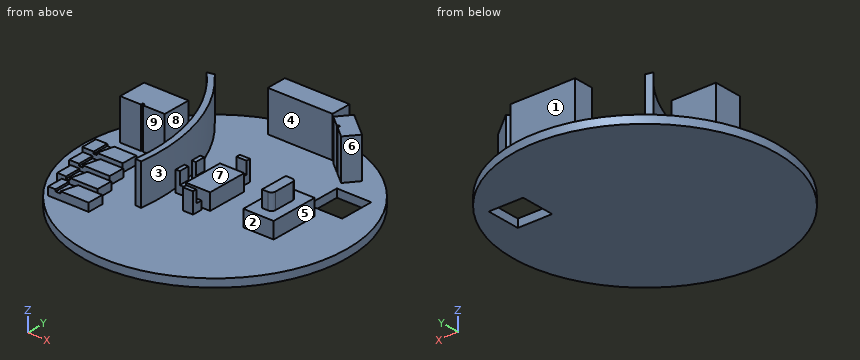
```python
from build123d import *

# Parameters (mm, degrees)
F0_R      = 32.5
F1_DEPTH  = 2
F2_W      = 16
F2_H      = 5
F3_DEPTH  = 10
F4_W      = 6
F4_H      = 10
F4_W_2    = 7.5
F4_H_2    = 12
F5_DEPTH  = 4
F6_W      = 2.5
F6_H      = 7
F7_DEPTH  = 4
F8_R      = 1
F9_W      = 2.5
F9_H      = 2.5
F10_DEPTH = 2
F11_W     = 2.5
F11_H     = 1
F11_W_2   = 1
F11_H_2   = 2.5
F12_DEPTH = 3
F13_W     = 8.5
F13_H     = 8.5
F14_DEPTH = 25
F15_W     = 10
F15_H     = 4
F16_DEPTH = 1.5
F17_W     = 2.795801
F17_H     = 4
F17_W_2   = 2.404703
F17_W_3   = 2.193978
F17_W_4   = 1.803281
F18_DEPTH = 0.5


with BuildPart() as f1:
    # F0 (on Top) → F1 (new body)
    with BuildSketch(Plane.XY):
        Circle(F0_R)
    extrude(amount=F1_DEPTH)

    # F2 (on face) → F3 (join)
    with BuildSketch(Plane.XY.offset(2)):
        with Locations((-0.270834, 27.762719)):
            Rectangle(F2_W, F2_H)
        Polygon((17.300418, 22.562942), (11.08706, 27.602206), (8.567428, 24.495527), (11.384874, 22.210474), (11.699828, 22.598809), (12.088162, 22.283855), (11.773208, 21.89552), (14.780786, 19.456263), align=None)
        Polygon((-16.460359, 11.750014), (-27.460359, 11.750014), (-27.460359, 4.750014), (-22.328375, 4.750014), (-22.328375, 5.250014), (-21.828375, 5.250014), (-21.828375, 4.750014), (-16.460359, 4.750014), align=None)
        with BuildLine():
            Line((-9.214541, -12.358905), (-7.719307, -12.482575))
            ThreePointArc((-7.719307, -12.482575), (-9.766223, 6.462552), (-19.395168, 22.906126))
            Line((-19.395168, 22.906126), (-21.053303, 22.485526))
            ThreePointArc((-21.053303, 22.485526), (-11.314103, 6.361134), (-9.214541, -12.358905))
        make_face()
    extrude(amount=F3_DEPTH)

    # F4 (on face) → F5 (join)
    with BuildSketch(Plane.XY.offset(2)):
        Rectangle(F4_W, F4_H)
        with Locations((15.75, 0.081453)):
            Rectangle(F4_W_2, F4_H_2)
    extrude(amount=F5_DEPTH)

    # F6 (on face) → F7 (join)
    with BuildSketch(Plane.XY.offset(6)):
        with Locations((15.75, 0.081453)):
            Rectangle(F6_W, F6_H)
    extrude(amount=F7_DEPTH)

    # F8
    f8_edges = [f1.edges().sort_by_distance(p)[0] for p in [
        (17, -3.418547, 8),
        (17, 3.581453, 8),
    ]]
    fillet(f8_edges, radius=F8_R)

    # F9 (on face) → F10 (join)
    with BuildSketch(Plane.XY.offset(2)):
        with Locations((-5.362472, -2.423183)):
            Rectangle(F9_W, F9_H)
        with Locations((-5.374835, 2.296795)):
            Rectangle(F9_W, F9_H)
        with Locations((0.118701, 7.372063)):
            Rectangle(F9_W, F9_H)
        with Locations((0.21179, -6.925349)):
            Rectangle(F9_W, F9_H)
    extrude(amount=F10_DEPTH)

    # F11 (on face) → F12 (join)
    with BuildSketch(Plane.XY.offset(4)):
        with Locations((0.21179, -7.675349)):
            Rectangle(F11_W, F11_H)
        with Locations((-6.124835, 2.296795)):
            Rectangle(F11_W_2, F11_H_2)
        with Locations((-6.112472, -2.423183)):
            Rectangle(F11_W_2, F11_H_2)
        with Locations((0.118701, 8.122063)):
            Rectangle(F11_W, F11_H)
    extrude(amount=F12_DEPTH)

    # F13 (on face) → F14 (cut)
    with BuildSketch(Plane.XY.offset(2)):
        with Locations((19.782292, 13.050183)):
            Rectangle(F13_W, F13_H)
    extrude(amount=-F14_DEPTH, mode=Mode.SUBTRACT)

    # F15 (on face) → F16 (join)
    with BuildSketch(Plane.XY.offset(2)):
        with Locations((-24.43407, -2)):
            Rectangle(F15_W, F15_H)
        with Locations((-23.044675, -7.475554)):
            Rectangle(F15_W, F15_H)
        with Locations((-21.457909, -12.888055)):
            Rectangle(F15_W, F15_H)
        with Locations((-19.281841, -18.088401)):
            Rectangle(F15_W, F15_H)
    extrude(amount=F16_DEPTH)

    # F17 (on face) → F18 (join)
    with BuildSketch(Plane.XY.offset(3.5)):
        with Locations((-28.036169, -2)):
            Rectangle(F17_W, F17_H)
        Polygon((-24.931015, 0), (-25.812697, -4), (-19.43407, -4), (-19.43407, 0), align=None)
        with Locations((-26.842323, -7.475554)):
            Rectangle(F17_W_2, F17_H)
        Polygon((-23.740886, -5.475554), (-24.701254, -9.475554), (-18.044675, -9.475554), (-18.044675, -5.475554), align=None)
        with Locations((-25.36092, -12.888055)):
            Rectangle(F17_W_3, F17_H)
        Polygon((-22.352759, -10.888055), (-23.25128, -14.888055), (-16.457909, -14.888055), (-16.457909, -10.888055), align=None)
        with Locations((-23.380201, -18.088401)):
            Rectangle(F17_W_4, F17_H)
        Polygon((-14.281841, -16.088401), (-20.255804, -16.088401), (-21.277487, -20.088401), (-14.281841, -20.088401), align=None)
    extrude(amount=F18_DEPTH)


solid = f1.part
```
The listing builds one solid part. Answer for the finished solid, in the listing's coordinates (mm). Face numbers are marked on the shaded views. A direction names the side the tool comes from. Give positions to 0.01 mm unless a question says otherwise; leave off trailing zeros. Loops run counter-clockwise (first coordinate to the right, second up) from the corner with the lowest first, then second, coordinate; pieces in that order, holes last. Notation, with made-up numbers: M 44.25,-12.75 L 52.25,-12.75 A24 cw 52.25,7.25 Z; hole C -15.5,-37 d4. An arc over 180 degrees is marked long. One line per item, written item: value.
1. Section B-B on y = 12.5 is taken. Determine the outline of the cut face in (x, z).
Found:
outline: M -30,0 L 15.53,0 L 15.53,2 L -12.25,2 L -12.25,12 L -13.93,12 L -13.93,2 L -30,2 Z; M 24.03,0 L 30,0 L 30,2 L 24.03,2 Z
2. Section D-D on x = 21 is taken. Determine the outline of the cut face in (y, z), plus the area to 3 significant figures.
Found:
outline: M -24.8,0 L 8.8,0 L 8.8,2 L -24.8,2 Z; M 17.3,0 L 24.8,0 L 24.8,2 L 17.3,2 Z
area: 82.2 mm^2
3. For the marked faces 1, 2, 3, 4 and 5, determine the directions among +Z, -Z, +X, -X, +Y, -Y from which every point of the face is accessible in a straight line to the end or side of a thin tool.
Found:
face 1: +Z, +X, -X, +Y
face 2: +Z, +X, -Y
face 3: +Z
face 4: +Z, -X
face 5: +Z, +X, +Y, -Y
4. For a pull along X with two mould halves and no side action, classify the marked faces 6, 7, 8 and 9 as pulls with the +X half, pulls with the -X half, needs draft (parallel to the pull), parting line crosses it, or undercut.
Found:
face 6: pulls with the +X half
face 7: undercut
face 8: undercut
face 9: needs draft
5. Section C-C on z = 8.75 is taken. State how many separate pieces and enclosed holes the cut face has, plus the area to 3 significant figures.
Found:
separate pieces: 5
enclosed holes: 0
area: 263 mm^2
6. Find the intervals of material crossed by probe 1 along Y at (x, z) = (0, 5.75); probe 2 along Y at (x, z) = (-6.5, 3.75); probe 3 along Y at (x, z) = (-23.5, 3), in increasing order.
Found:
probe 1: -8.18 to -7.18, -5 to 5, 7.62 to 8.62, 25.26 to 30.26
probe 2: -3.67 to -1.17, 1.05 to 3.55, 25.26 to 30.26
probe 3: -20.09 to -16.09, -14.89 to -10.89, -9.48 to -5.48, -4 to 0, 4.75 to 11.75
7. Section A-A on z = 1.25 is taken. Determine the outline of the cut face in (x, y), plus the area to 3 significant figures.
Found:
outline: C 0,0 d65; hole M 15.53,8.8 L 24.03,8.8 L 24.03,17.3 L 15.53,17.3 Z
area: 3,250 mm^2
8. Each of these flat-tipped pins is pushed along its axis until it touches: P1, Ø0.9, axis at x = -23, y = -18.5, coming from the +Z side; P2, Ø1, axis at y = -8.5, z = 3.5, coming from the +X side; P3, Ø1, axis at y = 12.5, z = 1, coming from the +X side. Where does it stop, or does it pass through?
Found:
P1: z = 4
P2: x = 1.46
P3: x = 30.2
